Autodesk Inventor part; units mm, degrees
ref_plane "YZ Plane" through (0, 0, 0) normal (1, 0, 0) x (0, 1, 0)
ref_plane "XZ Plane" through (0, 0, 0) normal (0, 1, 0) x (-1, 0, 0)
ref_plane "XY Plane" through (0, 0, 0) normal (0, 0, 1) x (1, 0, 0)
sketch "Sketch1" plane through (0, 0, 0) normal (0, 0, 1) x (1, 0, 0)
  line L0 (-12.7, -25.4) -> (12.7, -25.4)
  line L1 (12.7, -25.4) -> (12.7, 25.4)
  line L2 (12.7, 25.4) -> (-12.7, 25.4)
  line L3 (-12.7, 25.4) -> (-12.7, -25.4)
  line L4 (-12.7, -25.4) -> (12.7, 25.4) construction
  line L5 (12.7, -25.4) -> (-12.7, 25.4) construction
  line L6 (-11.1125, 23.8125) -> (11.1125, 23.8125)
  line L7 (11.1125, 23.8125) -> (11.1125, -23.8125)
  line L8 (11.1125, -23.8125) -> (-11.1125, -23.8125)
  line L9 (-11.1125, -23.8125) -> (-11.1125, 23.8125)
  point P0 (0, 0)
  dimension "width" = 25.4
  dimension "height" = 50.8
  dimension "thickness" = 1.5875
extrude "Extrusion1" add sketch "Sketch1" along normal mid plane 241.046
sketch "Sketch2" plane through (12.7, -25.4, 120.523) normal (1, 0, 0) x (0, 0, -1)
  line L0 (0, 49.2125) -> (0, 1.5875)
  line L1 (241.046, 50.8) -> (0, 50.8)
  line L2 (241.046, 50.8) -> (241.046, 0) construction
  point P0 (120.523, 25.4)
  point P1 (12.7, 38.1)
  point P2 (12.7, 12.7)
  point P3 (12.7, 25.4)
  point P4 (0, 25.4)
  point P5 (228.346, 38.1)
  point P6 (228.346, 12.7)
  point P7 (228.346, 25.4)
  point P8 (241.046, 25.4)
  dimension "d5" = 12.7
  dimension "d6" = 12.7
  dimension "d7" = 12.7
  dimension "d8" = 12.7
  dimension "d9" = 12.7
  dimension "d10" = 12.7
hole "Hole1" at (12.7, 12.7, 107.823) at (12.7, -12.7, 107.823) at (12.7, 0, 107.823) at (12.7, 12.7, -107.823) at (12.7, 0, -107.823) at (12.7, -12.7, -107.823) direction (-1, 0, 0) diameter 5.1054 end through all
sketch "Sketch3" plane through (-12.7, 25.4, 120.523) normal (0, 1, 0) x (1, 0, 0)
  line L0 (25.4, 0) -> (0, 0)
  line L1 (0, 241.046) -> (0, 0) construction
  line L2 (0, 241.046) -> (25.4, 241.046) construction
  point P0 (12.7, 120.523)
  point P1 (12.7, 6.35)
  point P2 (12.7, 12.7)
  point P3 (12.7, 19.05)
  point P4 (12.7, 234.696)
  point P5 (12.7, 228.346)
  point P6 (12.7, 221.996)
  dimension "d18" = 6.35
  dimension "d19" = 6.35
  dimension "d20" = 6.35
  dimension "d21" = 12.7
  dimension "d22" = 6.35
  dimension "d23" = 6.35
  dimension "d24" = 6.35
hole "Hole2" at (0, 25.4, 114.173) at (0, 25.4, 107.823) at (0, 25.4, 101.473) at (0, 25.4, -101.473) at (0, 25.4, -107.823) at (0, 25.4, -114.173) direction (0, -1, 0) diameter 5.1054 end through all
sketch "Sketch4" plane through (-12.7, 25.4, 120.523) normal (0, 1, 0) x (1, 0, 0)
  circle A0 centre (12.7, 228.346) radius 2.5527
  circle A1 centre (12.7, 19.05) radius 2.5527
  circle A2 centre (12.7, 6.35) radius 2.5527
  circle A3 centre (12.7, 12.7) radius 2.5527
  circle A4 centre (12.7, 221.996) radius 2.5527
  circle A5 centre (12.7, 234.696) radius 2.5527
  line L0 (0, 241.046) -> (25.4, 241.046)
  line L1 (25.4, 241.046) -> (25.4, 0)
  line L2 (25.4, 0) -> (0, 0)
  line L3 (0, 0) -> (0, 241.046)
  line L4 (6.35, 6.223) -> (19.05, 6.223) construction
  line L5 (19.05, 6.223) -> (19.05, 57.023) construction
  line L6 (19.05, 57.023) -> (6.35, 57.023) construction
  line L7 (6.35, 57.023) -> (6.35, 6.223) construction
  line L8 (6.35, 6.223) -> (19.05, 57.023) construction
  line L9 (19.05, 6.223) -> (6.35, 57.023) construction
  point P0 (12.7, 120.523)
  point P1 (12.7, 31.623)
  point P2 (12.7, 0)
  dimension "d32" = 12.7
  dimension "d33" = 50.8
  dimension "d34" = 31.623
hole "Hole3" at (-6.35, 25.4, 63.5) at (6.35, 25.4, 63.5) direction (0, -1, 0) diameter 5.1054 end through all
mirror "Mirror1" about plane through (0, 0, 0) normal (0, 0, 1) of "Hole3"
properties part number "EL2-006" material "Aluminum 6061"
CAD build for the part. Positions are in the model's coordinates, mm. Give positions to 0.01 mm unless a question says otherwise; leave off trailing zeros. Loops run counter-clockwise (first coordinate to the right, second up) from the corner with the lowest first, then second, coordinate; pieces in that order, holes last. Notation, with made-up numbers: (-2.75, -7.5) -> (11.25, -7.5) arc R20 cw to (11.25, -0.5) -> close; hole circle Ø9 at (77.5, 3.5). An arc over 180 degrees is marked (long way). Use a Markdown table: item, result.
1. Flat gauge pin, fed straight in: pin 1 (3 mm diameter, centred on x = 6.35, z = 63.5, fed in from +Y). Where does the tip first touch, or does it go through?
Check result:
| item | result |
|---|---|
| pin 1 | passes through |
2. Mould opens along Y. For faces 1 (the flat face through (0, -25.4, -2)), 2 (the flat face through (11.112, 0, -2)), 3 (the cylindrical face through (0.978, -24.617, -105.465)) say: pulls with the +Y half, pulls with the -Y half, needs draft (parallel to the pull), parting line crosses it, or undercut.
Check result:
| item | result |
|---|---|
| face 1 | pulls with the -Y half |
| face 2 | undercut |
| face 3 | needs draft |
3. Slice it at B-B (z = 63.5). List the corners of the cut face in (x, y).
Check result:
| item | result |
|---|---|
| outline | (-12.7, -25.4) -> (-8.9, -25.4) -> (-8.9, -23.81) -> (-11.11, -23.81) -> (-11.11, 23.81) -> (-8.9, 23.81) -> (-8.9, 25.4) -> (-12.7, 25.4) -> close; (-3.8, -25.4) -> (3.8, -25.4) -> (3.8, -23.81) -> (-3.8, -23.81) -> close; (-3.8, 23.81) -> (3.8, 23.81) -> (3.8, 25.4) -> (-3.8, 25.4) -> close; (8.9, -25.4) -> (12.7, -25.4) -> (12.7, 25.4) -> (8.9, 25.4) -> (8.9, 23.81) -> (11.11, 23.81) -> (11.11, -23.81) -> (8.9, -23.81) -> close |
4. Slice it at A-A (y = -12.7). List the corners of the cut face in (x, z).
Check result:
| item | result |
|---|---|
| outline | (-12.7, -120.52) -> (-11.11, -120.52) -> (-11.11, -110.38) -> (-12.7, -110.38) -> close; (-12.7, -105.27) -> (-11.11, -105.27) -> (-11.11, 105.27) -> (-12.7, 105.27) -> close; (-12.7, 110.38) -> (-11.11, 110.38) -> (-11.11, 120.52) -> (-12.7, 120.52) -> close; (11.11, -120.52) -> (12.7, -120.52) -> (12.7, -110.38) -> (11.11, -110.38) -> close; (11.11, -105.27) -> (12.7, -105.27) -> (12.7, 105.27) -> (11.11, 105.27) -> close; (11.11, 110.38) -> (12.7, 110.38) -> (12.7, 120.52) -> (11.11, 120.52) -> close |
5. Wall check: L1, parallel to Z at x = -11.9, y = 0; L2, parallel to X at y = -24.65, z = -63.5; L3, parallel to X at y = -19.5, z = -80. Give the ranges that are in metal, low to high. Write a range as [from, to].
Check result:
| item | result |
|---|---|
| L1 | z = [-120.52, -110.38], [-105.27, 105.27], [110.38, 120.52] |
| L2 | x = [-12.7, -8.9], [-3.8, 3.8], [8.9, 12.7] |
| L3 | x = [-12.7, -11.11], [11.11, 12.7] |
6. Slice it at D-D (z = 18). List the corners of the cut face in (x, y), plus the area to 3 significant figures.
Check result:
| item | result |
|---|---|
| outline | (-12.7, -25.4) -> (12.7, -25.4) -> (12.7, 25.4) -> (-12.7, 25.4) -> close; hole (-11.11, -23.81) -> (11.11, -23.81) -> (11.11, 23.81) -> (-11.11, 23.81) -> close |
| area | 232 mm^2 |
7. Slice it at C-C (x = -6.35). List the corners of the cut face in (y, z), plus the area to 3 significant figures.
Check result:
| item | result |
|---|---|
| outline | (-25.4, -120.52) -> (-23.81, -120.52) -> (-23.81, -66.05) -> (-25.4, -66.05) -> close; (-25.4, -60.95) -> (-23.81, -60.95) -> (-23.81, 60.95) -> (-25.4, 60.95) -> close; (-25.4, 66.05) -> (-23.81, 66.05) -> (-23.81, 120.52) -> (-25.4, 120.52) -> close; (23.81, -120.52) -> (25.4, -120.52) -> (25.4, -66.05) -> (23.81, -66.05) -> close; (23.81, -60.95) -> (25.4, -60.95) -> (25.4, 60.95) -> (23.81, 60.95) -> close; (23.81, 66.05) -> (25.4, 66.05) -> (25.4, 120.52) -> (23.81, 120.52) -> close |
| area | 733 mm^2 |
